For this review, take the finished solid that the model builds, in its own axes (mm). A direction names the side the tool comes from. Round coordinates to 2 decimals unless told otherwise and drop trailing zeros. Write each loop counter-clockwise with the first axis right and the second up, starting at its lowest first coordinate (ties: lowest second). Pieces come first, ordered by that corner, then holes. Notation, with made-up numbers: (-39, 57) -> (15, 57) arc R19 ccw to (15, 89) -> close; hole circle Ø11 at (47, 86.5). An arc over 180 degrees is marked (long way). Answer in a Markdown table with one row per item.
from build123d import *

# Parameters (mm, degrees)
REDONDEO1_R                = 2
TALADRO_ROSCADO_M64_D      = 5
TALADRO_ROSCADO_M64_DEPTH  = 18
TALADRO_ROSCADO_M64_TIP    = 1.502151548
TALADRO_ROSCADO_M69_D      = 5
TALADRO_ROSCADO_M69_DEPTH  = 18
TALADRO_ROSCADO_M69_TIP    = 1.502151548
TALADRO_ROSCADO_M611_D     = 5
TALADRO_ROSCADO_M611_DEPTH = 15
TALADRO_ROSCADO_M611_TIP   = 1.502151548
TALADRO_ROSCADO_M612_D     = 5
TALADRO_ROSCADO_M612_DEPTH = 15
TALADRO_ROSCADO_M612_TIP   = 1.502151548
TALADRO_ROSCADO_M613_D     = 5
TALADRO_ROSCADO_M613_DEPTH = 18
TALADRO_ROSCADO_M613_TIP   = 1.502151548
TALADRO_ROSCADO_M614_D     = 5
TALADRO_ROSCADO_M614_DEPTH = 18
TALADRO_ROSCADO_M614_TIP   = 1.502151548
TALADRO_ROSCADO_M615_D     = 5
TALADRO_ROSCADO_M615_DEPTH = 15
TALADRO_ROSCADO_M615_TIP   = 1.502151548


with BuildPart() as part:
    # Croquis1 → Revolución1 (revolve)
    with BuildSketch(Plane.XY, mode=Mode.PRIVATE) as revoluci_n1_sk:
        Polygon((0, 67), (70, 67), (70, 62), (64, 62), (64, 60), (12, 56), (12, 43), (64, 39), (64, 26), (49, 26), (49, 23), (25, 23), (25, 26), (10, 26), (10, 40), (0, 40), align=None)
    revolve(revoluci_n1_sk.sketch.rotate(Axis((-33.5154853, 0, 0), (1, 0, 0)), 90), axis=Axis((-33.5154853, 0, 0), (1, 0, 0)))

    # Redondeo1
    redondeo1_edges = [part.edges().sort_by_distance(p)[0] for p in [
        (12, 0, -43),
        (12, 0, -56),
    ]]
    fillet(redondeo1_edges, radius=REDONDEO1_R)

    # Taladro roscado M64
    with Locations(Plane(origin=(64, 0, 0), x_dir=(0, 0, -1), z_dir=(1, 0, 0))):
        with Locations((0, 32.5)):
            Hole(TALADRO_ROSCADO_M64_D / 2, depth=TALADRO_ROSCADO_M64_DEPTH)
            with Locations((0, 0, -(TALADRO_ROSCADO_M64_DEPTH + TALADRO_ROSCADO_M64_TIP / 2))):  # 118° drill point
                Cone(0, TALADRO_ROSCADO_M64_D / 2, TALADRO_ROSCADO_M64_TIP, mode=Mode.SUBTRACT)

    # Taladro roscado M69
    with Locations(Plane(origin=(64, 0, 0), x_dir=(0, 0, -1), z_dir=(1, 0, 0))):
        with Locations((0, -32.470562189)):
            Hole(TALADRO_ROSCADO_M69_D / 2, depth=TALADRO_ROSCADO_M69_DEPTH)
            with Locations((0, 0, -(TALADRO_ROSCADO_M69_DEPTH + TALADRO_ROSCADO_M69_TIP / 2))):  # 118° drill point
                Cone(0, TALADRO_ROSCADO_M69_D / 2, TALADRO_ROSCADO_M69_TIP, mode=Mode.SUBTRACT)

    # Taladro roscado M611
    with Locations(Plane.ZY.offset(-10)):
        with Locations((0, 32.498213501)):
            Hole(TALADRO_ROSCADO_M611_D / 2, depth=TALADRO_ROSCADO_M611_DEPTH)
            with Locations((0, 0, -(TALADRO_ROSCADO_M611_DEPTH + TALADRO_ROSCADO_M611_TIP / 2))):  # 118° drill point
                Cone(0, TALADRO_ROSCADO_M611_D / 2, TALADRO_ROSCADO_M611_TIP, mode=Mode.SUBTRACT)

    # Taladro roscado M612
    with Locations(Plane.ZY.offset(-10)):
        with Locations((0, -32.50019141)):
            Hole(TALADRO_ROSCADO_M612_D / 2, depth=TALADRO_ROSCADO_M612_DEPTH)
            with Locations((0, 0, -(TALADRO_ROSCADO_M612_DEPTH + TALADRO_ROSCADO_M612_TIP / 2))):  # 118° drill point
                Cone(0, TALADRO_ROSCADO_M612_D / 2, TALADRO_ROSCADO_M612_TIP, mode=Mode.SUBTRACT)

    # Taladro roscado M613
    with Locations(Plane(origin=(64, 0, 0), x_dir=(0, 0, -1), z_dir=(1, 0, 0))):
        with Locations((32.501693853, 0)):
            Hole(TALADRO_ROSCADO_M613_D / 2, depth=TALADRO_ROSCADO_M613_DEPTH)
            with Locations((0, 0, -(TALADRO_ROSCADO_M613_DEPTH + TALADRO_ROSCADO_M613_TIP / 2))):  # 118° drill point
                Cone(0, TALADRO_ROSCADO_M613_D / 2, TALADRO_ROSCADO_M613_TIP, mode=Mode.SUBTRACT)

    # Taladro roscado M614
    with Locations(Plane(origin=(64, 0, 0), x_dir=(0, 0, -1), z_dir=(1, 0, 0))):
        with Locations((32.5, 0), (-32.5, 0)):
            Hole(TALADRO_ROSCADO_M614_D / 2, depth=TALADRO_ROSCADO_M614_DEPTH)
            with Locations((0, 0, -(TALADRO_ROSCADO_M614_DEPTH + TALADRO_ROSCADO_M614_TIP / 2))):  # 118° drill point
                Cone(0, TALADRO_ROSCADO_M614_D / 2, TALADRO_ROSCADO_M614_TIP, mode=Mode.SUBTRACT)

    # Taladro roscado M615
    with Locations(Plane.ZY.offset(-10)):
        with Locations((-32.497793678, 0), (32.497518122, 0)):
            Hole(TALADRO_ROSCADO_M615_D / 2, depth=TALADRO_ROSCADO_M615_DEPTH)
            with Locations((0, 0, -(TALADRO_ROSCADO_M615_DEPTH + TALADRO_ROSCADO_M615_TIP / 2))):  # 118° drill point
                Cone(0, TALADRO_ROSCADO_M615_D / 2, TALADRO_ROSCADO_M615_TIP, mode=Mode.SUBTRACT)


solid = part.part
1) For faces 1 (the flat face through (49, 21, 10)), 2 (the flat face through (70, 59, 20)), 3 (the cylindrical face through (17.605, 0.11, 34.995)), list the 3-axis set-ups (+Z, -Z, +X, -X, +Y, -Y) from which the entire face can be reached by the end or side of a thin tool; tool diameter is ignored.
Solved:
| item | result |
|---|---|
| face 1 | +X |
| face 2 | +Z, -Z, +X, +Y, -Y |
| face 3 | -X |
2) For line 1 (Y direction, x = 29, z = 7.5); line 2 (Y direction, x = 41, z = 0); line 3 (Z direction, x = 14.5, y = -32), list the stretches that pass through material, from the lowest coordinate up. Write a range as [from, to].
Solved:
| item | result |
|---|---|
| line 1 | [-66.58, -56.81], [-41.01, -21.74], [21.74, 41.01], [56.81, 66.58] |
| line 2 | [-67, -58.23], [-40.77, -23], [23, 40.77], [58.23, 67] |
| line 3 | [-58.86, -46.19], [-28.43, -2.45], [2.45, 28.43], [46.19, 58.86] |
3) Consider section B-B on x = 30. State the section outline as (y, z) points.
Solved:
| item | result |
|---|---|
| outline | circle Ø134 at (0, 0); circle Ø83.23 at (0, 0); hole circle Ø114.77 at (0, 0); hole circle Ø46 at (0, 0) |
4) Consider section D-D on x = 8. State the section outline as (y, z) points, then the cut area to 3 significant figures.
Solved:
| item | result |
|---|---|
| outline | circle Ø134 at (0, 0); hole circle Ø80 at (0, 0) |
| area | 9,080 mm² |
5) Clearance check with flat-ended pins moving along their axes: pin 1 Ø4 at (x, z) = (45, 26.5) entering from +Y; pin 2 Ø3 at (x, z) = (43.5, 21.5) entering from +Y; pin 3 Ø6.5 at (y, z) = (-32.47, 0) entering from -X; pin 4 Ø10 at (y, z) = (-31.5, 36) entering from -X. State where each tip first meets the part, or that it passes through.
Solved:
| item | result |
|---|---|
| pin 1 | y = 62.36 |
| pin 2 | y = 63.95 |
| pin 3 | x = 10 |
| pin 4 | x = 0 |
6) Consider section C-C on x = 19. State the section outline as (y, z) points.
Solved:
| item | result |
|---|---|
| outline | circle Ø134 at (0, 0); circle Ø84.92 at (0, 0); hole circle Ø113.08 at (0, 0); hole circle Ø5 at (-32.5, 0); hole circle Ø52 at (0, 0); hole circle Ø5 at (0, -32.5); hole circle Ø5 at (0, 32.5); hole circle Ø5 at (32.5, 0) |
7) Mouldability with a two-part tool opening along Y and no side actions: class faces 4 (the flat face through (0, 29, -29)), 5 (the cylindrical face through (17.605, -0.958, -34.807)) as pulls with the +Y half, pulls with the -Y half, needs draft (parallel to the pull), parting line crosses it, or undercut.
Solved:
| item | result |
|---|---|
| face 4 | needs draft |
| face 5 | undercut |
8) Consider section A-A on x = 59.5. State the section outline as (y, z) points.
Solved:
| item | result |
|---|---|
| outline | circle Ø134 at (0, 0); circle Ø78.69 at (0, 0); hole circle Ø119.31 at (0, 0); hole circle Ø5 at (-32.47, 0); hole circle Ø52 at (0, 0); hole (-2.5, -32.5) arc R2.5 ccw to (2.5, -32.5) arc R2.5 ccw to start; hole circle Ø5 at (0, 32.5); hole circle Ø5 at (32.5, 0) |
